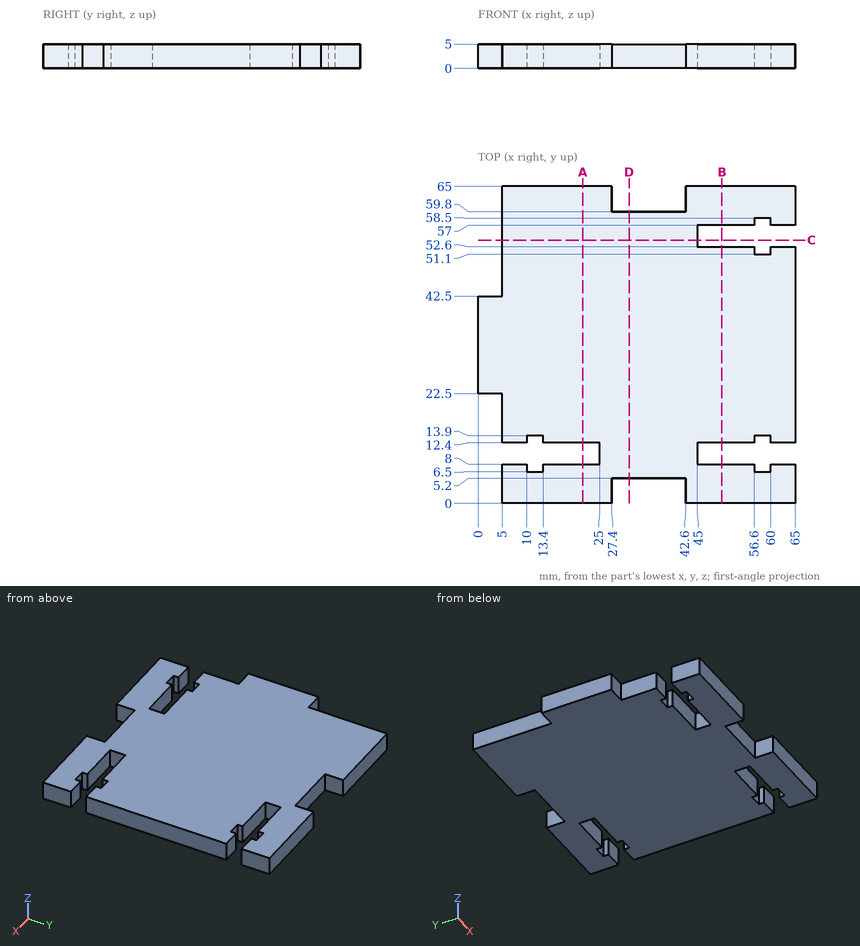
Can you work these out from the drawing? Everything is in mm from the part's minimum corner. Coordinates: 2 decimals unless noted, no trailing zeros. Loops run counter-clockwise (first coordinate to the right, second up) from the corner with the lowest first, then second, coordinate; pieces in that order, holes last.
1) Imagine slicing it at B-B on x = 50. List the corners of the cut face in (y, z) for me.
2) Imagine slicing it at A-A on x = 21.5. List the corners of the cut face in (y, z) for me.
3) Imagine slicing it at D-D on x = 31. List the corners of the cut face in (y, z) for me.
4) I need wall thicknesses on probe 1 along Y at (x, z) = (47.5, 1.2); probe 2 along Y at (x, z) = (23.5, 4.1); probe 3 along X at (y, z) = (58, 3.7). Which ranges of each line are inside material? Lowest first, please.
5) For pin 1 (1.5 mm diameter, centred on x = 2.5, z = 2, fed in from -Y); pin 2 (2 mm diameter, centred on x = 39, z = 1, fed in from -Y); pin 3 (2 mm diameter, centred on y = 9.5, z = 2, fed in from +X), each with a flat end and sliding along its axis, tell me the tip position at first contact or that it passes through.
6) Imagine slicing it at C-C on y = 54. List the corners of the cut face in (x, z) for me.
Completed:
1. outline: (0, 0) - (8, 0) - (8, 5) - (0, 5) - close; (12.4, 0) - (52.6, 0) - (52.6, 5) - (12.4, 5) - close; (57, 0) - (65, 0) - (65, 5) - (57, 5) - close
2. outline: (0, 0) - (8, 0) - (8, 5) - (0, 5) - close; (12.4, 0) - (65, 0) - (65, 5) - (12.4, 5) - close
3. outline: (5.2, 0) - (59.8, 0) - (59.8, 5) - (5.2, 5) - close
4. probe 1: y = 0 to 8, 12.4 to 52.6, 57 to 65
4. probe 2: y = 0 to 8, 12.4 to 65
4. probe 3: x = 5 to 56.6, 60 to 65
5. pin 1: stops at y = 22.5
5. pin 2: stops at y = 5.2
5. pin 3: stops at x = 45
6. outline: (5, 0) - (45, 0) - (45, 5) - (5, 5) - close
